The figure shows three views and two pictorial views of one solid part (mm, origin at its lowest corner). Answer the questions. Coordinates: 2 decimals unless noted, no trailing zeros. Write each loop counter-clockwise with the first axis right and the second up, starting at its lowest first coordinate (ties: lowest second). Pieces come first, ordered by that corner, then holes.
Item 1: Straight lines are drawn through the part: probe 1 along X at (y, z) = (4, 8.5); probe 2 along X at (y, z) = (11, 9.75); probe 3 along Y at (x, z) = (2.75, 7.75). For each, find the intervals that lie inside material, in ascending order.
Item 2: Section D-D (z = 8.5) is taken. Give the vertices of the cut face in (x, y).
Item 3: Section A-A (x = 9) is taken. Give the vertices of the cut face in (y, z), then the cut area to 3 significant figures.
Item 4: Section C-C (y = 8.5) is taken. Give the vertices of the cut face in (x, z), then the cut area to 3 significant figures.
Item 5: Section B-B (z = 1.75) is taken. Give the vertices of the cut face in (x, y), then the cut area to 3 significant figures.
Item 6: Determine the mould class of the marked faces 1, 2 and 3 for opening direction Z: released by +Z, released by -Z, zero draft, split by the parting line, or undercut.
Item 7: This flat-tipped pin is pushed along its axis until it touches: P1, Ø1, axis at x = 6, y = 7.5, coming from the +Z side. Where does it stop, or does it pass through?
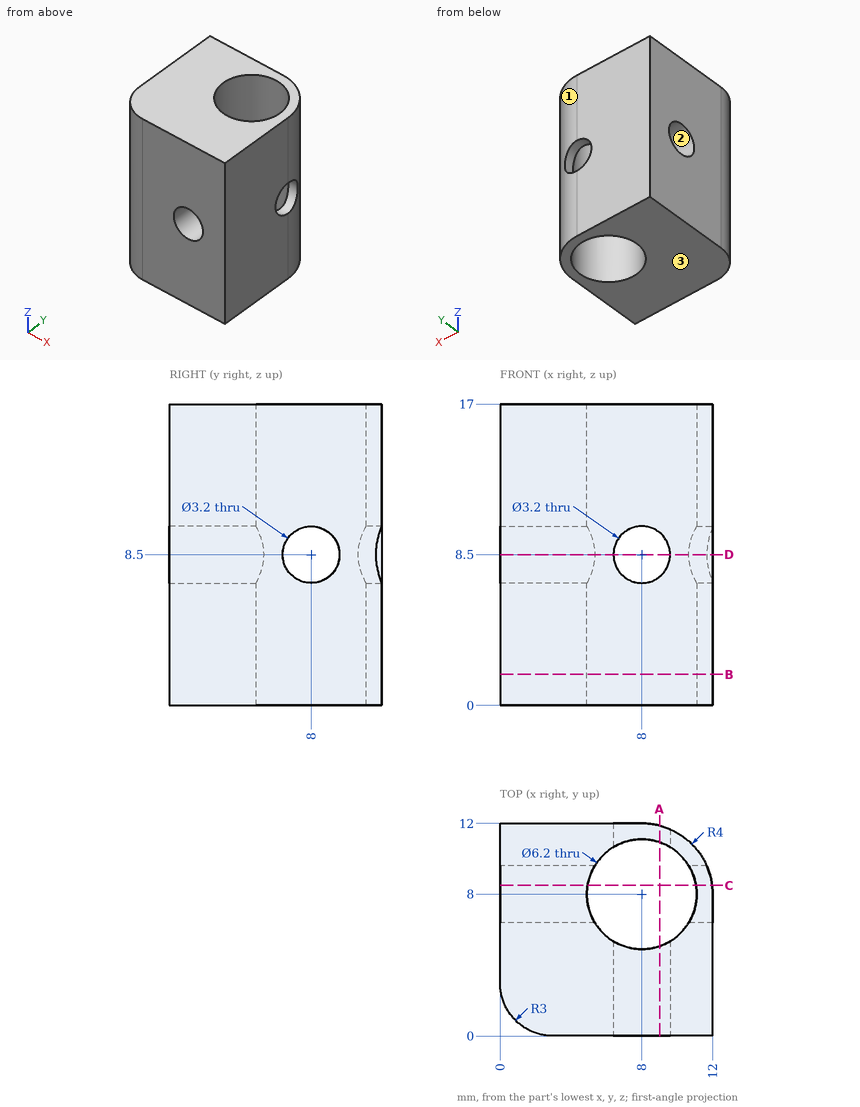
Established:
1. probe 1: x = 0 to 6.4, 9.6 to 12
1. probe 2: x = 0 to 7, 9 to 10.65
1. probe 3: y = 0.01 to 6.59, 9.41 to 12
2. outline: (0, 3) arc R3 ccw to (3, 0) - (6.4, 0) - (6.4, 5.34) arc R3.1 cw to (5.34, 6.4) - (0, 6.4) - close; (0, 9.6) - (5.34, 9.6) arc R3.1 cw to (6.4, 10.66) - (6.4, 12) - (0, 12) - close; (9.6, 0) - (12, 0) - (12, 6.4) - (10.66, 6.4) arc R3.1 cw to (9.6, 5.34) - close; (9.6, 10.66) arc R3.1 cw to (10.66, 9.6) - (11.67, 9.6) arc R4 ccw to (9.6, 11.67) - close
3. outline: (0, 0) - (5.07, 0) - (5.07, 7.25) - (0, 7.25) - close; (0, 9.75) - (5.07, 9.75) - (5.07, 17) - (0, 17) - close; (10.93, 0) - (11.87, 0) - (11.87, 7.25) - (10.93, 7.25) - close; (10.93, 9.75) - (11.87, 9.75) - (11.87, 17) - (10.93, 17) - close
3. area: 87.1 mm2
4. outline: (0, 0) - (4.94, 0) - (4.94, 6.98) - (0, 6.98) - close; (0, 10.02) - (4.94, 10.02) - (4.94, 17) - (0, 17) - close; (11.06, 0) - (11.97, 0) - (11.97, 6.98) - (11.06, 6.98) - close; (11.06, 10.02) - (11.97, 10.02) - (11.97, 17) - (11.06, 17) - close
4. area: 81.7 mm2
5. outline: (0, 3) arc R3 ccw to (3, 0) - (12, 0) - (12, 8) arc R4 ccw to (8, 12) - (0, 12) - close; hole circle Ø6.2 at (8, 8)
5. area: 108 mm2
6. face 1: zero draft
6. face 2: undercut
6. face 3: released by -Z
7. P1: passes through
